Design review of the part built by this model. Coordinates are the model's own, in mm. A direction names the side the tool comes from. Coordinates: 2 decimals unless noted, no trailing zeros. Loops run counter-clockwise (first coordinate to the right, second up) from the corner with the lowest first, then second, coordinate; pieces in that order, holes last. Notation, with made-up numbers: (81, -24.75) - (94, -24.75) arc R16 cw to (94, -19.75) - close; hole circle Ø4 at (29.25, 31.25). An arc over 180 degrees is marked (long way). One line per question, with ' | ' between items.
from build123d import *

# Parameters (mm, degrees)
F1_DEPTH = 50


with BuildPart() as f1:
    # F0 (on Front) → F1 (new body, symmetric)
    with BuildSketch(Plane.XZ):
        Polygon((2.5, -8.212121), (0, -8.212121), (-2.5, -8.212121), (-2.5, -4.212121), (-21.5, 14.787879), (-24, 14.787879), (-30, 8.787879), (-30, -8.212121), (-25, -8.212121), (-25, -28.212121), (-15, -28.212121), (-15, -23.212121), (0, -23.212121), (15, -23.212121), (15, -28.212121), (25, -28.212121), (25, -8.212121), (30, -8.212121), (30, 8.787879), (24, 14.787879), (21.5, 14.787879), (2.5, -4.212121), align=None)
    extrude(amount=F1_DEPTH, both=True)


solid = f1.part
Q1. Take a section at A-A (z = -6.5). Give the boundary of the cut face in (x, y), plus the area to 3 significant figures.
Returned:
outline: (-30, -50) - (-2.5, -50) - (-2.5, 50) - (-30, 50) - close; (2.5, -50) - (30, -50) - (30, 50) - (2.5, 50) - close | area: 5,500 mm²
Q2. Take a section at B-B (y = -19.5). Give the boundary of the cut face in (x, z), plus the area to 3 significant figures.
Returned:
outline: (-30, -8.21) - (-25, -8.21) - (-25, -28.21) - (-15, -28.21) - (-15, -23.21) - (15, -23.21) - (15, -28.21) - (25, -28.21) - (25, -8.21) - (30, -8.21) - (30, 8.79) - (24, 14.79) - (21.5, 14.79) - (2.5, -4.21) - (2.5, -8.21) - (-2.5, -8.21) - (-2.5, -4.21) - (-21.5, 14.79) - (-24, 14.79) - (-30, 8.79) - close | area: 1,720 mm²
Q3. To check wall thickness, follow line 1 along X through (y, z) = (23, -7.5); line 2 along X through (y, z) = (-40, -13); line 3 along X through (y, z) = (-14, 1). State the ranges of each line that lie inside material, in increasing order.
Returned:
line 1: x = -30 to -2.5, 2.5 to 30 | line 2: x = -25 to 25 | line 3: x = -30 to -7.71, 7.71 to 30
Q4. Draft analysis for pull direction X (two halves, no side actions). For faces 5 (the flat face through (20, -1, -28.212)), 6 (the flat face through (0, -1, -8.212)), 7 (the flat face through (-26.96, -0.7, 11.83)), 8 (the flat face through (-2.5, -1, -6)), state which applies: +X half, -X half, draft (parallel to the pull), parting line (faces both ways), or undercut.
Returned:
face 5: draft | face 6: undercut | face 7: -X half | face 8: undercut
Q5. Take a section at D-D (x = -17). Give the boundary of the cut face in (y, z), plus the area to 3 significant figures.
Returned:
outline: (-50, -28.21) - (50, -28.21) - (50, 10.29) - (-50, 10.29) - close | area: 3,850 mm²
Q6. For pin 1 (2.5 mm diameter, centred on y = -11.5, z = -25, fed in from -X); pin 2 (2.5 mm diameter, centred on x = 0, y = -9.5, fed in from +Z); pin 3 (5 mm diameter, centred on x = 5.5, y = 22, fed in from +Z), all flat-tipped, find the tip position at first contact; note any pin that passes through.
Returned:
pin 1: stops at x = -25 | pin 2: stops at z = -8.21 | pin 3: stops at z = 1.29
Q7. Take a section at C-C (z = 6.5). Give the boundary of the cut face in (x, y).
Returned:
outline: (-30, -50) - (-13.21, -50) - (-13.21, 50) - (-30, 50) - close; (13.21, -50) - (30, -50) - (30, 50) - (13.21, 50) - close
Q8. Tool access review of faces 1 (the flat face through (-28, -1, -8.212)), 2 (the flat face through (15, -1, -26)), 3 (the flat face through (-11.867, -0.7, 5.155)), 4 (the flat face through (27, -1, -8.212)): name each direction out of +Z, -Z, +X, -X, +Y, -Y from which nothing blocks a thin tool from reaching the whole face with its end or side.
Returned:
face 1: -Z, -X, +Y, -Y | face 2: -Z, +Y, -Y | face 3: +Z, +Y, -Y | face 4: -Z, +X, +Y, -Y
